Geometry check sheet. Reference: the model listing, model coordinates, mm. Face numbers are marked on the shaded views. A direction names the side the tool comes from. Give positions to 0.01 mm unless a question says otherwise; leave off trailing zeros. Loops run counter-clockwise (first coordinate to the right, second up) from the corner with the lowest first, then second, coordinate; pieces in that order, holes last. Notation, with made-up numbers: (68, 14) -> (72, 14) arc R31 cw to (72, 45) -> close; hole circle Ø4 at (86, -10). An arc over 180 degrees is marked (long way). Write each question's results on one line, items separated by ' | '. Start each with the question number.
1) Sectioned sample at B-B on z = 17.5. Record the cut outline in (x, y).
2) Sectioned sample at D-D on x = -11. Record the cut outline in (y, z).
3) Scan lines: line 1 (Y direction, x = 0, z = 26); line 2 (Z direction, x = 0, y = -15); line 3 (Z direction, x = -3.5, y = 0). Record each from-to range of solid material in increasing order. Write a range as from..to.
4) Set-up check for the marked faces 4, 5, 6 and 7: record each of +Z, -Z, +X, -X, +Y, -Y from which the full face is reachable in a straight line by a thin tool's end or side.
5) Sectioned sample at C-C on y = 17. Record the cut outline in (x, z).
6) Draft check along Y on the marked faces 1, 2 and 3. Enter one of: pulls with the +Y half, pulls with the -Y half, needs draft (parallel to the pull), parting line crosses it, or undercut.
7) Depth check by flat-ended pin: pin 1 (21.5 mm diameter, centred on y = -13.5, z = 7.5, fed in from +X); pin 2 (5 mm diameter, centred on y = -5.5, z = 21, fed in from -X); pin 3 (2.5 mm diameter, centred on x = 0.5, z = 27, fed in from +Y). Enter the tip coordinate at first touch or a pass-through.
8) Sectioned sample at A-A on x = 0. Record the cut outline in (y, z), then the cut area to 3 significant figures.
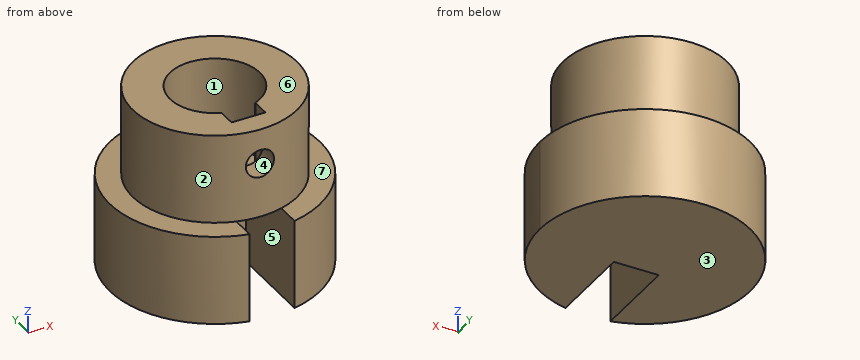
```python
from build123d import *

# Parameters (mm, degrees)
SALIENTE_EXTRUIR1_DEPTH = 20
CROQUIS2_R              = 18.253461236
SALIENTE_EXTRUIR2_DEPTH = 20
CROQUIS3_R              = 10
CROQUIS3_W              = 7.547979368
CROQUIS3_H              = 3.978601063
CORTAR_EXTRUIR1_DEPTH   = 20
CROQUIS4_R              = 3.130594147
CORTAR_EXTRUIR2_DEPTH   = 20


with BuildPart() as part:
    # Croquis1 → Saliente-Extruir1 (new body)
    with BuildSketch(Plane.XY):
        with BuildLine():
            Line((-5, -22.8595713), (-5, -3.514210375))
            Line((-5, -3.514210375), (5, -3.514210375))
            Line((5, -3.514210375), (5, -22.8595713))
            ThreePointArc((5, -22.8595713), (18.228549037, -14.672423113), (23.4, 0))
            ThreePointArc((23.4, 0), (-14.672423113, 18.228549037), (-5, -22.8595713))
        make_face()
    extrude(amount=SALIENTE_EXTRUIR1_DEPTH)

    # Croquis2 → Saliente-Extruir2 (add)
    with BuildSketch(Plane.XY.offset(20)):
        with Locations(Location((0, 0, 0), (0, 0, 254.102297609))):
            Circle(CROQUIS2_R)
    extrude(amount=SALIENTE_EXTRUIR2_DEPTH)

    # Croquis3 → Cortar-Extruir1 (cut)
    with BuildSketch(Plane.XY.offset(40)):
        Circle(CROQUIS3_R)
        with Locations((0.081314891, -11.282532094)):
            Rectangle(CROQUIS3_W, CROQUIS3_H)
    extrude(amount=-CORTAR_EXTRUIR1_DEPTH, mode=Mode.SUBTRACT)

    # Croquis4 → Cortar-Extruir2 (cut)
    with BuildSketch(Plane(origin=(0, 0, 0), x_dir=(1, 0, 0), z_dir=(0, 1, 0))):
        with Locations(Location((0, -32.173004338, 0), (0, 0, 270))):
            Circle(CROQUIS4_R)
    extrude(amount=-CORTAR_EXTRUIR2_DEPTH, mode=Mode.SUBTRACT)


solid = part.part
```
Result:
1) outline: (-5, -22.86) -> (-5, -3.51) -> (5, -3.51) -> (5, -22.86) arc R23.4 ccw (long way) to start
2) outline: (-20.65, 0) -> (20.65, 0) -> (20.65, 20) -> (14.57, 20) -> (14.57, 40) -> (-14.57, 40) -> (-14.57, 20) -> (-20.65, 20) -> close
3) line 1: -18.25..-13.27, 10..18.25 | line 2: 20..29.04, 35.3..40 | line 3: 0..20
4) face 4: -Y | face 5: -Z, -Y | face 6: +Z, +X, -X, +Y, -Y | face 7: +Z
5) outline: (-16.08, 0) -> (16.08, 0) -> (16.08, 20) -> (6.65, 20) -> (6.65, 40) -> (-6.65, 40) -> (-6.65, 20) -> (-16.08, 20) -> close
6) face 1: undercut | face 2: parting line crosses it | face 3: needs draft
7) pin 1: x = 23.24 | pin 2: x = -23.18 | pin 3: y = 18.25
8) outline: (-18.25, 20) -> (-13.27, 20) -> (-13.27, 29.04) -> (-18.25, 29.04) -> close; (-18.25, 35.3) -> (-13.27, 35.3) -> (-13.27, 40) -> (-18.25, 40) -> close; (-3.51, 0) -> (23.4, 0) -> (23.4, 20) -> (18.25, 20) -> (18.25, 40) -> (10, 40) -> (10, 20) -> (-3.51, 20) -> close | area: 772 mm^2
